For this review, take the finished solid that the model builds, in its own axes (mm). A direction names the side the tool comes from. Coordinates: 2 decimals unless noted, no trailing zeros. Loops run counter-clockwise (first coordinate to the right, second up) from the corner with the lowest first, then second, coordinate; pieces in that order, holes last. Notation, with made-up numbers: M -31,-29.5 L -1,-29.5 A8 cw -1,-25.5 Z; hole C -19,75 d2. An arc over 180 degrees is marked long. Answer as a JSON object with one key per item and string values. Group by question number.
Item 1: Add section A-A (z = -31). State the section outline as (x, y) points, then the cut area to 3 significant figures.
Item 2: Add section C-C (z = -54). State the section outline as (x, y) points.
Item 3: Add section B-B (y = 5.5). State the section outline as (x, z) points, then the cut area to 3 significant figures.
Item 4: Insertion check: pin 1 (7 mm diameter, centred on x = -80.48, z = -54, fed in from +Y); pin 2 (1.5 mm diameter, centred on y = 53, z = -55, fed in from +X); pin 3 (11.5 mm diameter, centred on x = -58, z = -36, fed in from +Y); pin 4 (2.5 mm diameter, centred on y = 53, z = -7.5, fed in from +X). Each pin has a flat end and moves straight along its axis. Give the tip position at first contact, or say it passes through.
Item 5: Add section D-D (x = -47.5). State the section outline as (y, z) points, then the cut area to 3 significant figures.
Item 6: Tool access review of faces 5 (the face through (-72.48, 51, -31)), 6 (the face through (-87.091, 39.293, -30.566)), 7 (the face through (-62.5, 54, -56)): name each direction out of +Z, -Z, +X, -X, +Y, -Y from which nothing blocks a thin tool from reaching the whole face with its end or side.
Item 7: Mouldability with a two-part tool opening along Z and no side actions: class faces 1 (the face through (-51, 46, 0)), 2 (the face through (-51, 50, -12)), 3 (the face through (-5, 8, -49)), 4 (the face through (-5, 0, -6)) as +Z half, -Z half, draft (parallel to the pull), parting line (faces both ways), or undercut.
Item 8: Wall thickness on L1, parallel to X at y = 8.5, z = -11.5; L2, parallel to Z at x = -70, y = 47.5; L3, parallel to Y at x = -30, z = -14.5: over which ranges is each line inside the solid? List them lowest first. Write a range as from..to.
from build123d import *

# Parameters (mm, degrees)
SCHIZZO1_W                   = 101
SCHIZZO1_H                   = 55
ESTRUSIONE_ESTRUSIONE1_DEPTH = 62
TAGLIO_ESTRUSIONE1_DEPTH     = 131.652210085
TAGLIO_ESTRUSIONE2_DEPTH     = 131.652210085
TAGLIO_ESTRUSIONE4_DEPTH     = 131.652210085
SCHIZZO8_W                   = 24
SCHIZZO8_H                   = 62
TAGLIO_ESTRUSIONE5_DEPTH     = 3
SCHIZZO9_W                   = 43.960031948
SCHIZZO9_H                   = 38
TAGLIO_ESTRUSIONE6_DEPTH     = 8
SCHIZZO10_R                  = 12
TAGLIO_ESTRUSIONE7_DEPTH     = 128.491176165
SCHIZZO11_R                  = 4
TAGLIO_ESTRUSIONE8_DEPTH     = 131.652210085


with BuildPart() as part:
    # Schizzo1 → Estrusione-Estrusione1 (new body)
    with BuildSketch(Plane.XY):
        with Locations((-50.5, 27.5)):
            Rectangle(SCHIZZO1_W, SCHIZZO1_H)
    extrude(amount=-ESTRUSIONE_ESTRUSIONE1_DEPTH)

    # Schizzo2 → Taglio-Estrusione1 (cut, through all)
    with BuildSketch(Plane(origin=(0, 0, 0), x_dir=(0, 0, -1), z_dir=(1, 0, 0))):
        with BuildLine():
            Line((13, 0), (49, 0))
            Line((49, 0), (49, 17))
            ThreePointArc((49, 17), (31, 29.91723747), (13, 17))
            Line((13, 17), (13, 0))
        make_face()
    extrude(amount=-TAGLIO_ESTRUSIONE1_DEPTH, mode=Mode.SUBTRACT)

    # Schizzo3 → Taglio-Estrusione2 (cut, through all)
    with BuildSketch(Plane.XY):
        with BuildLine():
            Line((-91, 0), (-10, 0))
            Line((-10, 0), (-10, 30))
            ThreePointArc((-10, 30), (-13.807611845, 39.192388155), (-23, 43))
            Line((-23, 43), (-78, 43))
            ThreePointArc((-78, 43), (-87.192388155, 39.192388155), (-91, 30))
            Line((-91, 30), (-91, 0))
        make_face()
    extrude(amount=-TAGLIO_ESTRUSIONE2_DEPTH, mode=Mode.SUBTRACT)

    # Schizzo7 → Taglio-Estrusione4 (cut, through all)
    with BuildSketch(Plane.XY):
        with BuildLine():
            Line((0, 55), (0, 30))
            ThreePointArc((0, 30), (-1.980372958, 39.751757321), (-7.607741667, 47.958545322))
            ThreePointArc((-7.607741667, 47.958545322), (-10.661934927, 51.062047082), (-12.519984026, 55))
            Line((-12.519984026, 55), (0, 55))
        make_face()
        with BuildLine():
            Line((-101, 55), (-101, 30))
            ThreePointArc((-101, 30), (-99.019627042, 39.751757321), (-93.392258333, 47.958545322))
            ThreePointArc((-93.392258333, 47.958545322), (-90.338065073, 51.062047082), (-88.480015974, 55))
            Line((-88.480015974, 55), (-101, 55))
        make_face()
    extrude(amount=-TAGLIO_ESTRUSIONE4_DEPTH, mode=Mode.SUBTRACT)

    # Schizzo8 → Taglio-Estrusione5 (cut)
    with BuildSketch(Plane(origin=(0, 55, 0), x_dir=(1, 0, 0), z_dir=(0, 1, 0))):
        with Locations((-50.5, 31)):
            Rectangle(SCHIZZO8_W, SCHIZZO8_H)
    extrude(amount=-TAGLIO_ESTRUSIONE5_DEPTH, mode=Mode.SUBTRACT)

    # Schizzo9 → Taglio-Estrusione6 (cut)
    with BuildSketch(Plane(origin=(0, 55, 0), x_dir=(1, 0, 0), z_dir=(0, 1, 0))):
        with Locations((-50.5, 31)):
            Rectangle(SCHIZZO9_W, SCHIZZO9_H)
    extrude(amount=-TAGLIO_ESTRUSIONE6_DEPTH, mode=Mode.SUBTRACT)

    # Schizzo10 → Taglio-Estrusione7 (cut, through all)
    with BuildSketch(Plane(origin=(0, 47, 0), x_dir=(1, 0, 0), z_dir=(0, 1, 0))):
        with Locations(Location((-50.5, 31, 0), (0, 0, 270))):
            Circle(SCHIZZO10_R)
    extrude(amount=-TAGLIO_ESTRUSIONE7_DEPTH, mode=Mode.SUBTRACT)

    # Schizzo11 → Taglio-Estrusione8 (cut, through all)
    with BuildSketch(Plane(origin=(0, 55, 0), x_dir=(1, 0, 0), z_dir=(0, 1, 0))):
        with Locations(Location((-80.480015974, 54, 0), (0, 0, 180))):
            Circle(SCHIZZO11_R)
        with Locations(Location((-20.480015974, 54, 0), (0, 0, 180))):
            Circle(SCHIZZO11_R)
        with Locations(Location((-20.480015974, 8, 0), (0, 0, 180))):
            Circle(SCHIZZO11_R)
        with Locations(Location((-80.480015974, 8, 0), (0, 0, 180))):
            Circle(SCHIZZO11_R)
    extrude(amount=-TAGLIO_ESTRUSIONE8_DEPTH, mode=Mode.SUBTRACT)


solid = part.part
From the geometry:
{
 "1": {"outline": "M -101,29.92 L -91,29.92 L -91,30 A13 cw -78,43 L -62.5,43 L -62.5,47 L -72.48,47 L -72.48,55 L -88.48,55 A13 cw -93.39,47.96 A25 ccw -101,30 Z; M -38.5,43 L -23,43 A13 cw -10,30 L -10,29.92 L 0,29.92 L 0,30 A25 ccw -7.61,47.96 A13 cw -12.52,55 L -28.52,55 L -28.52,47 L -38.5,47 Z", "area": "864 mm²"},
 "2": {"outline": "M -101,0 L -91,0 L -91,30 A13 cw -84.48,41.27 L -84.48,55 L -88.48,55 A13 cw -93.39,47.96 A25 ccw -101,30 Z; M -76.48,43 L -24.48,43 L -24.48,55 L -38.5,55 L -38.5,52 L -62.5,52 L -62.5,55 L -76.48,55 Z; M -16.48,41.25 A13 cw -10,30 L -10,0 L 0,0 L 0,30 A25 ccw -7.61,47.96 A13 cw -12.52,55 L -16.48,55 Z"},
 "3": {"outline": "M -101,-62 L -91,-62 L -91,-49 L -101,-49 Z; M -101,-13 L -91,-13 L -91,0 L -101,0 Z; M -10,-62 L 0,-62 L 0,-49 L -10,-49 Z; M -10,-13 L 0,-13 L 0,0 L -10,0 Z", "area": "520 mm²"},
 "4": {"pin 1": "passes through", "pin 2": "stops at x = -11.4", "pin 3": "stops at y = 47", "pin 4": "stops at x = -11.11"},
 "5": {"outline": "M 43,-62 L 52,-62 L 52,-50 L 47,-50 L 47,-42.62 L 43,-42.62 Z; M 43,-19.38 L 47,-19.38 L 47,-12 L 52,-12 L 52,0 L 43,0 Z", "area": "275 mm²"},
 "6": {"face 5": "+Y", "face 6": "+Z, -Z, -Y", "face 7": "+Z, -Z, +Y"},
 "7": {"face 1": "+Z half", "face 2": "undercut", "face 3": "undercut", "face 4": "draft"},
 "8": {"L1": "x = -101..-91, -10..0", "L2": "z = -62..-50, -12..0", "L3": "y = 43..47"}
}
